Source: CAD feature listing. Evaluate the final solid. Frame: model axes, mm. A direction names the side the tool comes from. Round coordinates to 2 decimals unless told otherwise and drop trailing zeros. Order: outer loops, then holes, each group sorted by start corner. A loop starts at its lowest first (then second) coordinate and runs counter-clockwise, first axis right, second up. Notation, with made-up numbers: (-8.75, 37.25) -> (13.25, 37.25) arc R21 ccw to (13.25, 69.25) -> close; hole circle Ø10 at (88, 37.25). An arc over 180 degrees is marked (long way). One line per item, written item: value. Start each with the question number.
1) Reachability of faces 1 (the face through (20, 39.497, 1)), 2 (the face through (41, 58.697, 1)) from +Z, -Z, +X, -X, +Y, -Y: full face, straight path, thin tool, end or side. Return the list, or none.
2) Section C-C (z = 0.7). State how many separate pieces and enclosed holes the cut face has, and give its area (3 significant figures).
3) Pin query (flat end, axial travel): P1, Ø1.5, axis at x = 57, y = 52, coming from the +Z side. Return the tip coordinate at first contact, or that it passes through.
4) Ray query, L1, parallel to Y at x = 44, z = 0.1; L2, parallel to Y at x = 57.5, z = 1.4; L3, parallel to X at y = 19, z = 1. Return the intervals inside material, ascending.
5) Section B-B (y = 45). Return the cut outline in (x, z), and give its area (3 significant figures).
6) Section A-A (x = 37). Return the cut outline in (y, z), and give its area (3 significant figures).
```python
from build123d import *

# Parameters (mm, degrees)
F0_W      = 57
F0_H      = 57
F1_DEPTH  = 1.6
F4_R      = 0.5
F5_R      = 0.5
F6_R      = 0.5
F2_R      = 0.5
F7_DEPTH  = 4
F8_R      = 3
F9_R      = 1
F10_DEPTH = 25
F12_DEPTH = 5
F13_W     = 4
F13_H     = 1.7
F14_DEPTH = 25
F15_R     = 0.2


with BuildPart() as f1:
    # F0 (on Top) → F1 (new body)
    with BuildSketch(Plane.XY):
        with Locations((41.31729, 30.19701)):
            Rectangle(F0_W, F0_H)
    extrude(amount=F1_DEPTH)

    # F4 (on face) + F5 (on face) + F6 (on face) + F3 (on face) + F2 (on face) → F7 (cut)
    with BuildSketch(Plane.XY.offset(1.6)):
        with Locations((51.61729, 22.19701)):
            Circle(F4_R)
        with Locations((56.61729, 22.19701)):
            Circle(F4_R)
        with Locations((54.11729, 22.19701)):
            Circle(F4_R)
    with BuildSketch(Plane.XY.offset(1.6)):
        with Locations((40.06729, 30.69701)):
            Circle(F5_R)
        with Locations((42.56729, 30.69701)):
            Circle(F5_R)
    with BuildSketch(Plane.XY.offset(1.6)):
        with Locations((27.56729, 22.19701)):
            Circle(F6_R)
        with Locations((31.06729, 22.19701)):
            Circle(F6_R)
    with BuildSketch(Plane.XY.offset(1.6)):
        with BuildLine():
            ThreePointArc((53.81729, 31.34701), (53.56729, 31.09701), (53.81729, 30.84701))
            Line((53.81729, 30.84701), (54.81729, 30.84701))
            ThreePointArc((54.81729, 30.84701), (55.06729, 31.09701), (54.81729, 31.34701))
            Line((54.81729, 31.34701), (53.81729, 31.34701))
        make_face()
        with BuildLine():
            ThreePointArc((51.86729, 28.69701), (52.11729, 28.94701), (51.86729, 29.19701))
            Line((51.86729, 29.19701), (51.16729, 29.19701))
            ThreePointArc((51.16729, 29.19701), (50.91729, 28.94701), (51.16729, 28.69701))
            Line((51.16729, 28.69701), (51.86729, 28.69701))
        make_face()
        with BuildLine():
            Line((56.76729, 28.69701), (57.46729, 28.69701))
            ThreePointArc((57.46729, 28.69701), (57.71729, 28.94701), (57.46729, 29.19701))
            Line((57.46729, 29.19701), (56.76729, 29.19701))
            ThreePointArc((56.76729, 29.19701), (56.51729, 28.94701), (56.76729, 28.69701))
        make_face()
    with BuildSketch(Plane.XY.offset(1.6)):
        with Locations((27.31729, 30.19701)):
            Circle(F2_R)
        with Locations((29.31729, 30.19701)):
            Circle(F2_R)
        with Locations((31.31729, 30.19701)):
            Circle(F2_R)
    extrude(amount=-F7_DEPTH, mode=Mode.SUBTRACT)

    # F8
    f8_edges = [f1.edges().sort_by_distance(p)[0] for p in [
        (12.81729, 1.69701, 0.8),
        (69.81729, 1.69701, 0.8),
        (69.81729, 58.69701, 0.8),
        (12.81729, 58.69701, 0.8),
    ]]
    fillet(f8_edges, radius=F8_R)

    # F9 (on face) → F10 (cut)
    with BuildSketch(Plane.XY.offset(1.6)):
        with Locations((63.31729, 24.69701)):
            Circle(F9_R)
        with Locations((19.31729, 24.69701)):
            Circle(F9_R)
        with Locations((55.31729, 37.29701)):
            Circle(F9_R)
        with Locations((27.31729, 37.29701)):
            Circle(F9_R)
        with Locations((15.31729, 56.19701)):
            Circle(F9_R)
        with Locations((67.31729, 56.19701)):
            Circle(F9_R)
        with Locations((15.31729, 4.19701)):
            Circle(F9_R)
        with Locations((67.31729, 4.19701)):
            Circle(F9_R)
        with Locations((41.31729, 56.19701)):
            Circle(F9_R)
        with Locations((41.31729, 4.19701)):
            Circle(F9_R)
        with Locations((15.31729, 30.19701)):
            Circle(F9_R)
        with Locations((67.31729, 30.19701)):
            Circle(F9_R)
    extrude(amount=-F10_DEPTH, mode=Mode.SUBTRACT)

    # F11 (on face) → F12 (cut)
    with BuildSketch(Plane.XY.offset(1.6)):
        with BuildLine():
            ThreePointArc((66.81729, 19.19701), (66.670844, 19.550563), (66.31729, 19.69701))
            Line((66.31729, 19.69701), (16.31729, 19.69701))
            ThreePointArc((16.31729, 19.69701), (15.963737, 19.550563), (15.81729, 19.19701))
            Line((15.81729, 19.19701), (15.81729, 7.19701))
            ThreePointArc((15.81729, 7.19701), (15.963737, 6.843456), (16.31729, 6.69701))
            Line((16.31729, 6.69701), (66.31729, 6.69701))
            ThreePointArc((66.31729, 6.69701), (66.670844, 6.843456), (66.81729, 7.19701))
            Line((66.81729, 7.19701), (66.81729, 19.19701))
        make_face()
        with BuildLine():
            ThreePointArc((16.31729, 53.69701), (15.963737, 53.550563), (15.81729, 53.19701))
            Line((15.81729, 53.19701), (15.81729, 41.19701))
            ThreePointArc((15.81729, 41.19701), (15.963737, 40.843456), (16.31729, 40.69701))
            Line((16.31729, 40.69701), (66.31729, 40.69701))
            ThreePointArc((66.31729, 40.69701), (66.670844, 40.843456), (66.81729, 41.19701))
            Line((66.81729, 41.19701), (66.81729, 53.19701))
            ThreePointArc((66.81729, 53.19701), (66.670844, 53.550563), (66.31729, 53.69701))
            Line((66.31729, 53.69701), (16.31729, 53.69701))
        make_face()
    extrude(amount=-F12_DEPTH, mode=Mode.SUBTRACT)

    # F13 (on face) → F14 (cut)
    with BuildSketch(Plane.XY.offset(1.6)):
        with Locations((19.533351, 4.64701)):
            Rectangle(F13_W, F13_H)
        with Locations((63.101229, 4.64701)):
            Rectangle(F13_W, F13_H)
        with Locations((63.101229, 21.74701)):
            Rectangle(F13_W, F13_H)
        with Locations((19.533351, 21.74701)):
            Rectangle(F13_W, F13_H)
        with Locations((19.533351, 38.64701)):
            Rectangle(F13_W, F13_H)
        with Locations((19.533351, 55.74701)):
            Rectangle(F13_W, F13_H)
        with Locations((63.101229, 38.64701)):
            Rectangle(F13_W, F13_H)
        with Locations((63.101229, 55.74701)):
            Rectangle(F13_W, F13_H)
    extrude(amount=-F14_DEPTH, mode=Mode.SUBTRACT)

    # F15
    f15_edges = [f1.edges().sort_by_distance(p)[0] for p in [
        (17.533351, 56.59701, 0.8),
        (17.533351, 54.89701, 0.8),
        (21.533351, 54.89701, 0.8),
        (21.533351, 56.59701, 0.8),
        (21.533351, 39.49701, 0.8),
        (17.533351, 39.49701, 0.8),
        (17.533351, 37.79701, 0.8),
        (21.533351, 37.79701, 0.8),
        (65.101229, 54.89701, 0.8),
        (65.101229, 56.59701, 0.8),
        (61.101229, 56.59701, 0.8),
        (61.101229, 54.89701, 0.8),
        (61.101229, 37.79701, 0.8),
        (61.101229, 39.49701, 0.8),
        (65.101229, 39.49701, 0.8),
        (65.101229, 37.79701, 0.8),
        (21.533351, 20.89701, 0.8),
        (21.533351, 22.59701, 0.8),
        (17.533351, 22.59701, 0.8),
        (17.533351, 20.89701, 0.8),
        (61.101229, 20.89701, 0.8),
        (61.101229, 22.59701, 0.8),
        (65.101229, 22.59701, 0.8),
        (65.101229, 20.89701, 0.8),
        (65.101229, 3.79701, 0.8),
        (65.101229, 5.49701, 0.8),
        (61.101229, 5.49701, 0.8),
        (61.101229, 3.79701, 0.8),
        (17.533351, 3.79701, 0.8),
        (21.533351, 3.79701, 0.8),
        (21.533351, 5.49701, 0.8),
        (17.533351, 5.49701, 0.8),
    ]]
    fillet(f15_edges, radius=F15_R)


solid = f1.part
```
Findings:
1. face 1: +Z, -Z
1. face 2: +Z, -Z, +X, -X, +Y
2. separate pieces: 1
2. enclosed holes: 35
2. area: 1,810 mm2
3. P1: through
4. L1: 1.7 to 6.7, 19.7 to 40.7, 53.7 to 58.7
4. L2: 1.7 to 6.7, 19.7 to 28.7, 29.19 to 40.7, 53.7 to 58.7
4. L3: 12.82 to 15.82, 66.82 to 69.82
5. outline: (12.82, 0) -> (15.82, 0) -> (15.82, 1.6) -> (12.82, 1.6) -> close; (66.82, 0) -> (69.82, 0) -> (69.82, 1.6) -> (66.82, 1.6) -> close
5. area: 9.60 mm2
6. outline: (1.7, 0) -> (6.7, 0) -> (6.7, 1.6) -> (1.7, 1.6) -> close; (19.7, 0) -> (40.7, 0) -> (40.7, 1.6) -> (19.7, 1.6) -> close; (53.7, 0) -> (58.7, 0) -> (58.7, 1.6) -> (53.7, 1.6) -> close
6. area: 49.6 mm2
